```python
from build123d import *

# Parameters (mm, degrees)
BOSS_EXTRUDE1_DEPTH = 5
SKETCH2_R           = 2
CUT_EXTRUDE1_DEPTH  = 203.531099834
SKETCH3_W           = 140.92
SKETCH3_H           = 25
BOSS_EXTRUDE2_DEPTH = 8
SKETCH4_R           = 2
CUT_EXTRUDE2_DEPTH  = 203.886289335
SKETCH5_R           = 4
CUT_EXTRUDE3_DEPTH  = 5
CHAMFER1_SIZE       = 10
CUT_EXTRUDE4_DEPTH  = 5
SKETCH8_R           = 2
CUT_EXTRUDE5_DEPTH  = 203.627358469


with BuildPart() as part:
    # Sketch1 → Boss-Extrude1 (new body)
    with BuildSketch(Plane(origin=(0, 0, 0), x_dir=(1, 0, 0), z_dir=(0, 1, 0))):
        Polygon((170.92, 20), (200.92, 20), (200.92, 0), (0, 0), (0, 20), (30, 20), (30, 25), (170.92, 25), align=None)
    extrude(amount=BOSS_EXTRUDE1_DEPTH)

    # Sketch2 → Cut-Extrude1 (cut, through all)
    with BuildSketch(Plane(origin=(0, 5, 0), x_dir=(1, 0, 0), z_dir=(0, 1, 0))):
        with Locations(Location((14, 10, 0), (0, 0, 270))):
            Circle(SKETCH2_R)
        with Locations(Location((186.92, 10, 0), (0, 0, 270))):
            Circle(SKETCH2_R)
    extrude(amount=-CUT_EXTRUDE1_DEPTH, mode=Mode.SUBTRACT)

    # Sketch3 → Boss-Extrude2 (add)
    with BuildSketch(Plane(origin=(0, 0, 0), x_dir=(1, 0, 0), z_dir=(0, 1, 0))):
        with Locations((100.46, 12.5)):
            Rectangle(SKETCH3_W, SKETCH3_H)
    extrude(amount=-BOSS_EXTRUDE2_DEPTH)

    # Sketch4 → Cut-Extrude2 (cut, through all)
    with BuildSketch(Plane(origin=(0, 5, 0), x_dir=(1, 0, 0), z_dir=(0, 1, 0))):
        with Locations(Location((70.46, 13, 0), (0, 0, 270))):
            Circle(SKETCH4_R)
        with Locations(Location((40.46, 13, 0), (0, 0, 270))):
            Circle(SKETCH4_R)
        with Locations(Location((160.46, 13, 0), (0, 0, 90))):
            Circle(SKETCH4_R)
        with Locations(Location((130.46, 13, 0), (0, 0, 90))):
            Circle(SKETCH4_R)
    extrude(amount=-CUT_EXTRUDE2_DEPTH, mode=Mode.SUBTRACT)

    # Sketch5 → Cut-Extrude3 (cut)
    with BuildSketch(Plane.XZ.offset(8)):
        with Locations(Location((40.46, -13, 0), (0, 0, 270))):
            Circle(SKETCH5_R)
        with Locations(Location((130.46, -13, 0), (0, 0, 270))):
            Circle(SKETCH5_R)
        with Locations(Location((160.46, -13, 0), (0, 0, 270))):
            Circle(SKETCH5_R)
        with Locations(Location((70.46, -13, 0), (0, 0, 270))):
            Circle(SKETCH5_R)
    extrude(amount=-CUT_EXTRUDE3_DEPTH, mode=Mode.SUBTRACT)

    # Chamfer1
    chamfer1_edges = [part.edges().sort_by_distance(p)[0] for p in [
        (200.92, 2.5, 0),
        (0, 2.5, 0),
    ]]
    chamfer(chamfer1_edges, length=CHAMFER1_SIZE)

    # Sketch6 → Cut-Extrude4 (cut)
    with BuildSketch(Plane.XZ.offset(8)):
        Polygon((92.46, 0), (108.46, 0), (108.46, -10.07179677), (104.46, -17), (96.46, -17), (92.46, -10.07179677), align=None)
    extrude(amount=-CUT_EXTRUDE4_DEPTH, mode=Mode.SUBTRACT)

    # Sketch8 → Cut-Extrude5 (cut, through all)
    with BuildSketch(Plane.XZ.offset(3)):
        with Locations(Location((100.46, -13, 0), (0, 0, 270))):
            Circle(SKETCH8_R)
    extrude(amount=-CUT_EXTRUDE5_DEPTH, mode=Mode.SUBTRACT)


solid = part.part
```
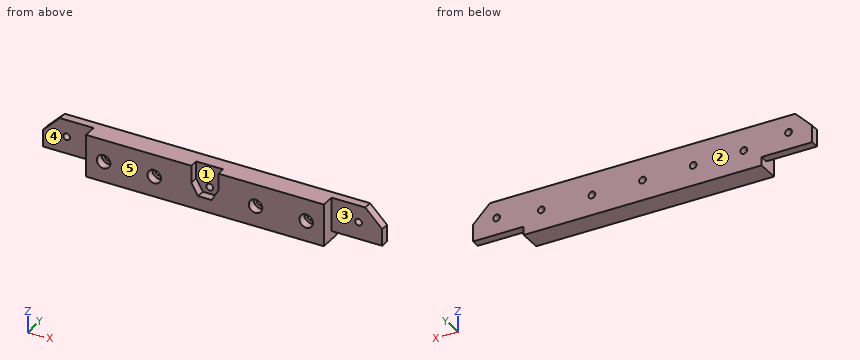
Could you check a few things on this model? Use its own coordinates, in mm. Face numbers are marked on the shaded views. A direction names the side the tool comes from. Coordinates: 2 decimals unless noted, no trailing zeros. Write each loop counter-clockwise with the first axis right and the second up, starting at its lowest first coordinate (ties: lowest second). Pieces come first, ordered by that corner, then holes. Notation, with made-up numbers: (64.5, 61.25) -> (93.5, 61.25) arc R9 ccw to (93.5, 67.25) -> close; hole circle Ø11 at (-25, -21.75). An arc over 180 degrees is marked (long way). Write item = value, one per line. Start each with the question number.
(1) I want a section at B-B (y = -6.25). Please give me the cut outline in (x, z), plus the area to 3 significant figures.
(2) I want a section at C-C (z = -4.75). Please give me the cut outline in (x, y).
(3) I want a section at D-D (x = 100.46). Please give me the cut outline in (y, z).
(4) Which directions (+Z, -Z, +X, -X, +Y, -Y) give clear straight access to the entire face, cutting with the end or side of a thin tool? Please do the marked faces 1, 2, 3, 4 and 5.
(5) I need wall thicknesses on line 1 (X direction, y = -0.25, z = -13); line 2 (X direction, y = -4.75, z = -6); line 3 (X direction, y = 1.85, z = -10). Which ranges of each line are inside material? Lowest first, please. Write a range as [from, to].
(6) Will these pins go through, and if not, where does the flat tip stop? pin 1 (2.5 mm diameter, centred on x = 99, y = -6, fed in from +Z); pin 2 (2.5 mm diameter, centred on x = 128.5, z = -14, fed in from -Y); pin 3 (1.5 mm diameter, centred on x = 27.5, y = 2.5, fed in from -Z).
(7) I want a section at A-A (x = 14). Please give me the cut outline in (y, z), plus the area to 3 significant figures.
Result set:
q1.outline = (30, -25) -> (170.92, -25) -> (170.92, 0) -> (108.46, 0) -> (108.46, -10.07) -> (104.46, -17) -> (96.46, -17) -> (92.46, -10.07) -> (92.46, 0) -> (30, 0) -> close; hole circle Ø8 at (40.46, -13); hole circle Ø8 at (70.46, -13); hole circle Ø8 at (130.46, -13); hole circle Ø8 at (160.46, -13)
q1.area = 3,080 mm2
q2.outline = (5.25, 0) -> (30, 0) -> (30, -8) -> (92.46, -8) -> (92.46, -3) -> (108.46, -3) -> (108.46, -8) -> (170.92, -8) -> (170.92, 0) -> (195.67, 0) -> (195.67, 5) -> (5.25, 5) -> close
q3.outline = (-8, -25) -> (5, -25) -> (5, -15) -> (-3, -15) -> (-3, -17) -> (-8, -17) -> close; (-3, -11) -> (5, -11) -> (5, 0) -> (-3, 0) -> close
q4.face_1 = +Z, -Y
q4.face_2 = +Z, -Z, +X, -X, +Y
q4.face_3 = +Z, -Z, +X, -Y
q4.face_4 = +Z, -Z, -X, -Y
q4.face_5 = +Z, -Z, +X, -X, -Y
q5.line_1 = [30, 38.46], [42.46, 68.46], [72.46, 98.46], [102.46, 128.46], [132.46, 158.46], [162.46, 170.92]
q5.line_2 = [30, 92.46], [108.46, 170.92]
q5.line_3 = [0, 12], [16, 184.92], [188.92, 200.92]
q6.pin_1 = -17
q6.pin_2 = -3
q6.pin_3 = -20
q7.outline = (0, -20) -> (5, -20) -> (5, -12) -> (0, -12) -> close; (0, -8) -> (5, -8) -> (5, 0) -> (0, 0) -> close
q7.area = 80.0 mm2
